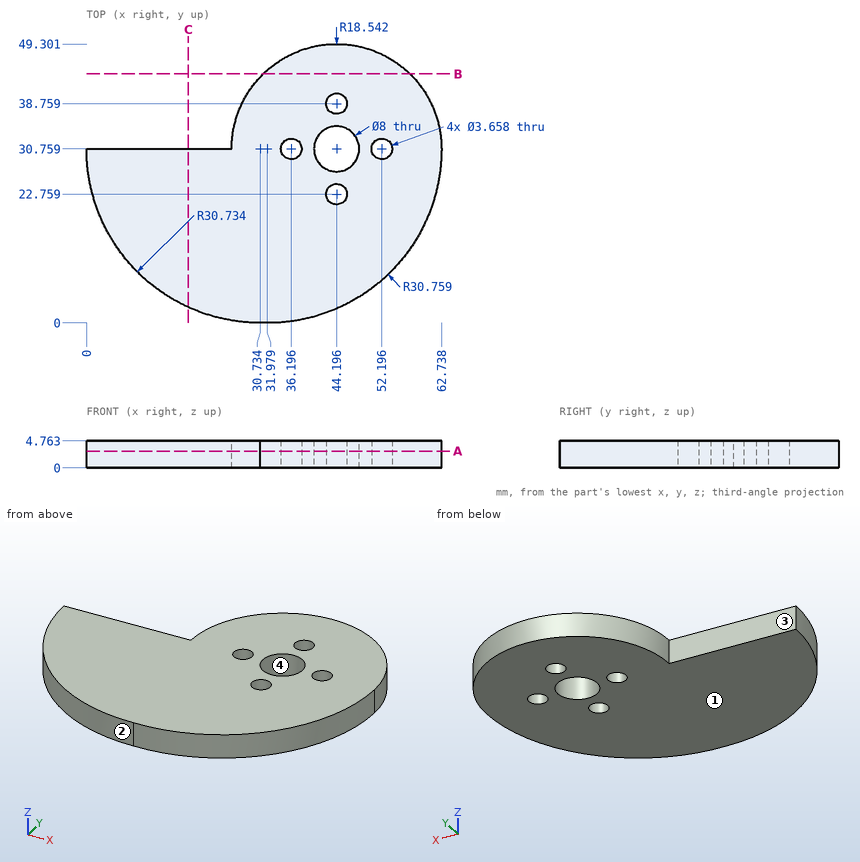
Design review of the part shown in the three views and the two pictorial views. Dimensions are in mm from the part's minimum x, y and z. Round coordinates to 2 decimals unless told otherwise and drop trailing zeros. Write each loop counter-clockwise with the first axis right and the second up, starting at its lowest first coordinate (ties: lowest second). Pieces come first, ordered by that corner, then holes.
Item 1: For probe 1 along Y at (x, z) = (44.5, 3.5) (1 decimal); probe 2 along X at (y, z) = (23.5, 3.05) (1 decimal); probe 3 along X at (y, z) = (28.5, 1.2) (1 decimal), list the stretches that pass through material, from the lowest coordinate up.
Item 2: We need section A-A on z = 2.95. Write out the cut boundary in (x, y) (1 decimal), and give its area (3 significant figures).
Item 3: We need section C-C on x = 18. Write out the cut boundary in (y, z), and give its area (3 significant figures).
Item 4: The part is to be moulded in two halves that separate along Y. For the marked faces 1, 2, 3 and 4, say which applies: +Y half, -Y half, draft (parallel to the pull), parting line (faces both ways), or undercut.
Item 5: Clearance check with flat-ended pins moving along their axes: pin 1 Ø1.5 at (y, z) = (41.5, 2.5) entering from -X (1 decimal); pin 2 Ø1 at (x, z) = (28, 0.5) entering from -Y; pin 3 Ø3.5 at (x, y) = (44.2, 38.76) entering from +Z; pin 4 Ø1.4 at (x, z) = (10.5, 1.5) entering from +Y. State where each tip first meets the part, or that it passes through.
Item 6: We need section B-B on y = 44. Write out the cut boundary in (x, z) (1 decimal), and give its area (3 significant figures).
Returned:
1. probe 1: y = 2.7 to 21, 24.6 to 26.8, 34.7 to 37, 40.6 to 49.3
1. probe 2: x = 0.9 to 42.5, 45.9 to 61.9
1. probe 3: x = 0.1 to 40.9, 47.5 to 62.7
2. outline: (0, 30.8) arc R30.7 ccw to (30.7, 0) arc R30.8 ccw to (62.7, 30.8) arc R18.5 ccw to (25.7, 30.8) - close; hole circle Ø3.7 at (36.2, 30.8); hole circle Ø8 at (44.2, 30.8); hole circle Ø3.7 at (44.2, 22.8); hole circle Ø3.7 at (44.2, 38.8); hole circle Ø3.7 at (52.2, 30.8)
2. area: 1,970 mm2
3. outline: (2.79, 0) - (30.76, 0) - (30.76, 4.76) - (2.79, 4.76) - close
3. area: 133 mm2
4. face 1: draft
4. face 2: -Y half
4. face 3: +Y half
4. face 4: undercut
5. pin 1: stops at x = 28.6
5. pin 2: stops at y = 0.11
5. pin 3: passes through
5. pin 4: stops at y = 30.76
6. outline: (31.2, 0) - (57.2, 0) - (57.2, 4.8) - (31.2, 4.8) - close
6. area: 124 mm2
